Geometry check sheet. Reference: the model listing, model coordinates, mm. A direction names the side the tool comes from. Coordinates: 2 decimals unless noted, no trailing zeros. Write each loop counter-clockwise with the first axis right and the second up, starting at its lowest first coordinate (ties: lowest second). Pieces come first, ordered by that corner, then holes.
from build123d import *

# Parameters (mm, degrees)
BOSS_EXTRUDE1_DEPTH = 1
SKETCH2_R           = 2.35
CUT_EXTRUDE1_DEPTH  = 32.4
LPATTERN1_COUNT     = 2
LPATTERN1_PITCH     = 2


with BuildPart() as part:
    # Sketch1 → Revolve1 (revolve)
    with BuildSketch(Plane(origin=(0, 0, 0), x_dir=(1, 0, 0), z_dir=(0, 1, 0))):
        with BuildLine():
            Line((-18.91291866, 0), (13.48708134, 0))
            Line((13.48708134, 0), (13.48708134, -3.25))
            Line((13.48708134, -3.25), (9.986643337, -3.867221664))
            ThreePointArc((9.986643337, -3.867221664), (9.660069022, -3.77971634), (9.517184066, -3.473298563))
            Line((9.517184066, -3.473298563), (9.517184066, -3.415711135))
            Line((9.517184066, -3.415711135), (6.956540611, -3.867221664))
            ThreePointArc((6.956540611, -3.867221664), (6.629966296, -3.77971634), (6.48708134, -3.473298563))
            Line((6.48708134, -3.473298563), (6.48708134, -3.421019058))
            Line((6.48708134, -3.421019058), (3.956540611, -3.867221664))
            ThreePointArc((3.956540611, -3.867221664), (3.629966296, -3.77971634), (3.48708134, -3.473298563))
            Line((3.48708134, -3.473298563), (3.48708134, -3.25))
            Line((3.48708134, -3.25), (-14.943021387, -3.25))
            Line((-14.943021387, -3.25), (-14.943021387, -3.473298563))
            ThreePointArc((-14.943021387, -3.473298563), (-15.085906343, -3.77971634), (-15.412480658, -3.867221664))
            Line((-15.412480658, -3.867221664), (-18.91291866, -3.25))
            Line((-18.91291866, -3.25), (-18.91291866, 0))
        make_face()
    revolve(axis=Axis((-25.423923445, 0, 0), (1, 0, 0)))

    # Sketch3 → Boss-Extrude1 (add)
    with BuildSketch(Plane(origin=(-7.443021387, 0, 0), x_dir=(0, 0, -1), z_dir=(1, 0, 0))):
        with BuildLine():
            Line((4.5, -4.5), (-4.5, -4.5))
            Line((-4.5, -4.5), (-4.5, 0))
            ThreePointArc((-4.5, 0), (0, 4.5), (4.5, 0))
            Line((4.5, 0), (4.5, -4.5))
        make_face()
    boss_extrude1 = extrude(amount=BOSS_EXTRUDE1_DEPTH)

    # Sketch2 → Cut-Extrude1 (cut)
    with BuildSketch(Plane(origin=(13.48708134, 0, 0), x_dir=(0, 0, -1), z_dir=(1, 0, 0))):
        Circle(SKETCH2_R)
    extrude(amount=-CUT_EXTRUDE1_DEPTH, mode=Mode.SUBTRACT)

    # LPattern1: Boss-Extrude1 ×2
    with Locations(*[(i * LPATTERN1_PITCH, 0, 0) for i in range(1, LPATTERN1_COUNT)]):
        add(boss_extrude1)


solid = part.part
1. Thickness scan on line 1 along X through (y, z) = (1.5, -3.75); line 2 along Y through (x, z) = (-11.25, 0); line 3 along X through (y, z) = (2, 0.75). Record the ranges inside material, lowest first.
Computed values:
line 1: x = -7.44 to -6.44, -5.44 to -4.44
line 2: y = -3.25 to -2.35, 2.35 to 3.25
line 3: x = -5.44 to -4.44
2. Gauge pin test, flat ends, axial feed: pin 1 Ø4 at (y, z) = (-1, -0.5) entering from -X; pin 2 Ø2 at (x, z) = (-9.5, 3) entering from -Y; pin 3 Ø1.5 at (x, y) = (-8, 1) entering from +Z; pin 4 Ø4 at (x, y) = (4, 3) entering from +Z. Record the tip position at first contact, or that the pin passes through.
Computed values:
pin 1: stops at x = -18.91
pin 2: stops at y = -2.56
pin 3: stops at z = 4.47
pin 4: stops at z = 3.74
3. Sectioned sample at B-B, the plane x = 5.5. Record the boundary of the cut face in (y, z), and give its area (3 significant figures).
Computed values:
outline: circle Ø7.19 at (0, 0); hole circle Ø4.7 at (0, 0)
area: 23.3 mm2
4. Sectioned sample at A-A, the plane x = -9.5. Record the boundary of the cut face in (y, z), and give its area (3 significant figures).
Computed values:
outline: circle Ø6.5 at (0, 0); hole circle Ø4.7 at (0, 0)
area: 15.8 mm2
5. Draft check along Y on faces 4 (the flat face through (-5, -4.5, 0)), 5 (the cylindrical face through (-11.246, 1.978, -2.579)), 6 (the cylindrical face through (-12.084, -2.294, 0.509)). Enter one of: released by +Y, released by -Y, zero draft, split by the parting line, or undercut.
Computed values:
face 4: released by -Y
face 5: split by the parting line
face 6: undercut
6. Access from +Z, -Z, +X, -X, +Y, -Y to the whole of each face (thin tool, end or side, straight path). Record for faces 1 (the flat face through (-4.443, 0, 0)), 2 (the cylindrical face through (-0.533, 1.978, -2.579)), 3 (the conical face through (-17.965, -3.388, -0.445)).
Computed values:
face 1: +X
face 2: none
face 3: -X
